Could you check a few things on this drawing? It's one solid part, dimensions in mm from its lowest x, y, z. A direction names the side the tool comes from. Round coordinates to 2 decimals unless told otherwise and drop trailing zeros. Write each loop counter-clockwise with the first axis right and the second up, starting at its lowest first coordinate (ties: lowest second). Pieces come first, ordered by that corner, then holes. Notation, with made-up numbers: (-33, 16) -> (19, 16) arc R24 ccw to (19, 27) -> close; hole circle Ø2 at (2.25, 47.5). An arc over 180 degrees is marked (long way). Return JSON: item names as keys, results as strings.
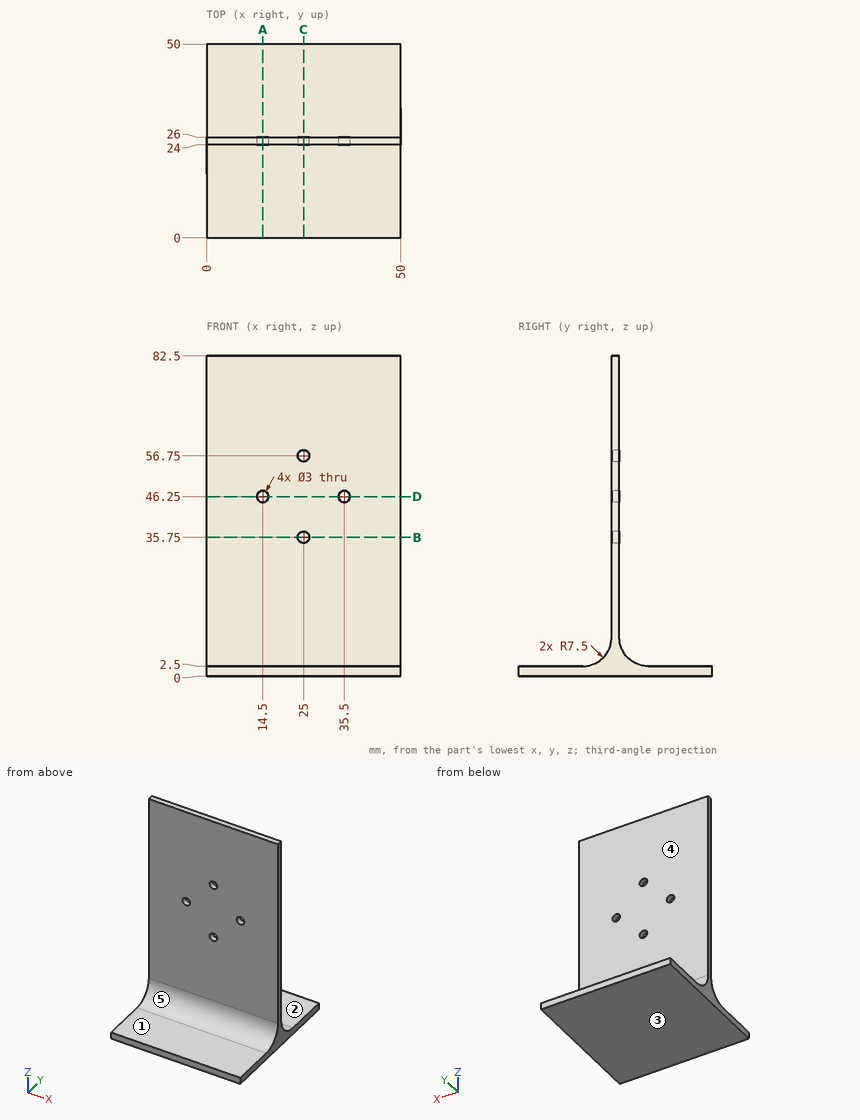
1) For the marked faces 1 and 2, which set-ups out of +Z, -Z, +X, -X, +Y, -Y let a thin tool reach every point of the face, with its end or its side?
Return value:
{"face 1": "+Z, +X, -X, -Y", "face 2": "+Z, +X, -X, +Y"}
2) I want a section at B-B, the plane z = 35.75. Please give me the cut outline in (x, y).
Return value:
{"outline": "(0, 24) -> (23.5, 24) -> (23.5, 26) -> (0, 26) -> close; (26.5, 24) -> (50, 24) -> (50, 26) -> (26.5, 26) -> close"}
3) I want a section at D-D, the plane z = 46.25. Please give me the cut outline in (x, y).
Return value:
{"outline": "(0, 24) -> (13, 24) -> (13, 26) -> (0, 26) -> close; (16, 24) -> (34, 24) -> (34, 26) -> (16, 26) -> close; (37, 24) -> (50, 24) -> (50, 26) -> (37, 26) -> close"}
4) I want a section at A-A, the plane x = 14.5. Please give me the cut outline in (y, z).
Return value:
{"outline": "(0, 0) -> (50, 0) -> (50, 2.5) -> (33.5, 2.5) arc R7.5 cw to (26, 10) -> (26, 44.75) -> (24, 44.75) -> (24, 10) arc R7.5 cw to (16.5, 2.5) -> (0, 2.5) -> close; (24, 47.75) -> (26, 47.75) -> (26, 82.5) -> (24, 82.5) -> close"}
5) Will these pins go through, and if not, where does the flat tip stop? pin 1 Ø15 at (x, z) = (25.5, 62.5) entering from +Y; pin 2 Ø2.5 at (x, z) = (35.5, 46.25) entering from -Y; pin 3 Ø1 at (x, y) = (5, 13.5) entering from +Z; pin 4 Ø3.5 at (x, z) = (25, 56.75) entering from -Y.
Return value:
{"pin 1": "y = 26", "pin 2": "through", "pin 3": "z = 2.5", "pin 4": "y = 24"}
6) If I drill on probe 1 along Z at (x, y) = (25, 24.4); probe 2 along X at (y, z) = (25.5, 46.25); probe 3 along Z at (x, y) = (14.5, 24.9), over which ranges is the centre line in solid material (lowest first)? Write a range as [from, to].
Return value:
{"probe 1": "[0, 34.25], [37.25, 55.25], [58.25, 82.5]", "probe 2": "[0, 13], [16, 34], [37, 50]", "probe 3": "[0, 44.75], [47.75, 82.5]"}
7) Thinking about a two-plate mould opening in Z: for the marked faces 3, 4 and 5, which applies, pulls with the +Z half, pulls with the -Z half, needs draft (parallel to the pull), parting line crosses it, or undercut?
Return value:
{"face 3": "pulls with the -Z half", "face 4": "needs draft", "face 5": "pulls with the +Z half"}
8) I want a section at C-C, the plane x = 25. Please give me the cut outline in (y, z), and give its area (3 significant figures).
Return value:
{"outline": "(0, 0) -> (50, 0) -> (50, 2.5) -> (33.5, 2.5) arc R7.5 cw to (26, 10) -> (26, 34.25) -> (24, 34.25) -> (24, 10) arc R7.5 cw to (16.5, 2.5) -> (0, 2.5) -> close; (24, 37.25) -> (26, 37.25) -> (26, 55.25) -> (24, 55.25) -> close; (24, 58.25) -> (26, 58.25) -> (26, 82.5) -> (24, 82.5) -> close", "area": "297 mm²"}
